Check sheet for the modelled part. Datum: model origin and axes. Units: mm. A direction names the side the tool comes from. Coordinates: 2 decimals unless noted, no trailing zeros. Write each loop counter-clockwise with the first axis right and the second up, starting at its lowest first coordinate (ties: lowest second). Pieces come first, ordered by that corner, then holes. Notation, with made-up numbers: (-6.75, 42.5) -> (12.25, 42.5) arc R7 cw to (12.25, 53.5) -> close; hole circle Ø2 at (-35, -5.75). An arc over 180 degrees is marked (long way). Put each result on its own line as item: value.
```python
from build123d import *

# Parameters (mm, degrees)
SKETCH_1_W               = 800
SKETCH_1_H               = 2400
EXTRUDE_1_DEPTH          = 20
SKETCH_2_W               = 50
SKETCH_2_H               = 50
EXTRUDE_2_DEPTH          = 710
MIRROR_2_COPY_1_SKETCH_W = 50
MIRROR_2_COPY_1_SKETCH_H = 50
MIRROR_2_COPY_1_DEPTH    = 710


with BuildPart() as part:
    # 草图1 → 凸台-拉伸1 (new body)
    with BuildSketch(Plane(origin=(0, 0, 0), x_dir=(1, 0, 0), z_dir=(0, 1, 0))):
        Rectangle(SKETCH_1_W, SKETCH_1_H)
    extrude(amount=EXTRUDE_1_DEPTH)

    # 草图2 → 凸台-拉伸2 (add)
    with BuildSketch(Plane(origin=(0, 0, 0), x_dir=(-1, 0, 0), z_dir=(0, -1, 0))):
        with Locations((-375, -1175)):
            Rectangle(SKETCH_2_W, SKETCH_2_H)
    extrude_2 = extrude(amount=EXTRUDE_2_DEPTH)

    # 镜向1: 凸台-拉伸2 across plane
    add(extrude_2.mirror(Plane.XY))

    # 镜向2: 凸台-拉伸2 across plane
    add(extrude_2.mirror(Plane(origin=(0, 0, 0), x_dir=(0, 0, 1), z_dir=(1, 0, 0))))

    # 镜向2 copy 1 sketch → 镜向2 copy 1 (add)
    with BuildSketch(Plane.XZ):
        with Locations((-375, -1175)):
            Rectangle(MIRROR_2_COPY_1_SKETCH_W, MIRROR_2_COPY_1_SKETCH_H)
    extrude(amount=MIRROR_2_COPY_1_DEPTH)


solid = part.part
```
Q1. Material ranges on line 1 along Z through (x, y) = (-355.5, -510.5); line 2 along Y through (x, z) = (327, -240.5), recorded low to high.
Recorded:
line 1: z = -1200 to -1150, 1150 to 1200
line 2: y = 0 to 20
Q2. Cross-section at B-B (x = -262). Record the cut outline in (y, z), plus the area to 3 significant figures.
Recorded:
outline: (0, -1200) -> (20, -1200) -> (20, 1200) -> (0, 1200) -> close
area: 48,000 mm2
Q3. Tool access check on faces 1 (the flat face through (375, -350, 1150)), 2 (the flat face through (-375, -710, 1175)), 3 (the flat face through (-350, -350, -1175)). Record the directions out of +Z, -Z, +X, -X, +Y, -Y that give a thin tool (end or side, any length) a straight path to the whole face; none if there is none.
Recorded:
face 1: +X, -X, -Y
face 2: +Z, -Z, +X, -X, -Y
face 3: +Z, -Z, -Y
Q4. Depth check by flat-ended pin: P1, Ø12, axis at x = 9.5, z = -237.5, coming from the -Y side. Enter the tip coordinate at first touch or a pass-through.
Recorded:
P1: stops at y = 0
Q5. Cross-section at A-A (y = -635). Record the cut outline in (x, z), plus the area to 3 significant figures.
Recorded:
outline: (-400, -1200) -> (-350, -1200) -> (-350, -1150) -> (-400, -1150) -> close; (-400, 1150) -> (-350, 1150) -> (-350, 1200) -> (-400, 1200) -> close; (350, -1200) -> (400, -1200) -> (400, -1150) -> (350, -1150) -> close; (350, 1150) -> (400, 1150) -> (400, 1200) -> (350, 1200) -> close
area: 10,000 mm2
Q6. Mould release check, pull along X, two halves, no side actions. Record for faces 4 (the flat face through (400, 8, -539)), 5 (the flat face through (-350, -350, 1175)), 6 (the flat face through (-2, 8, -1200)): released by +X, released by -X, zero draft, split by the parting line, or undercut.
Recorded:
face 4: released by +X
face 5: undercut
face 6: zero draft
Q7. Cross-section at C-C (z = -704.5). Record the cut outline in (x, y), plus the area to 3 significant figures.
Recorded:
outline: (-400, 0) -> (400, 0) -> (400, 20) -> (-400, 20) -> close
area: 16,000 mm2
